Design review of the part built by this model. Coordinates are the model's own, in mm. Coordinates: 2 decimals unless noted, no trailing zeros. Write each loop counter-clockwise with the first axis right and the second up, starting at its lowest first coordinate (ties: lowest second). Pieces come first, ordered by that corner, then holes.
Q1. Add section A-A, the plane x = -51.5. Give the number of separate pieces and of enclosed holes in the cut face, plus the area to 3 significant figures.
Q2. To check wall thickness, follow probe 1 along Y at (x, z) = (-132.5, 1.15); probe 2 along X at (y, z) = (333.5, 0.15); probe 3 along Y at (x, z) = (132.5, 1.25). State the ranges of each line that lie inside material, in increasing order.
Q3. Add section C-C, the plane y = 200.5. Give the boundary of the cut face in (x, z).
Q4. Clearance check with a flat-ended pin moving along its axis: pin 1 Ø0.6 at (y, z) = (333, 1.5) entering from +X. State where the tip first meets the part, or that it passes through.
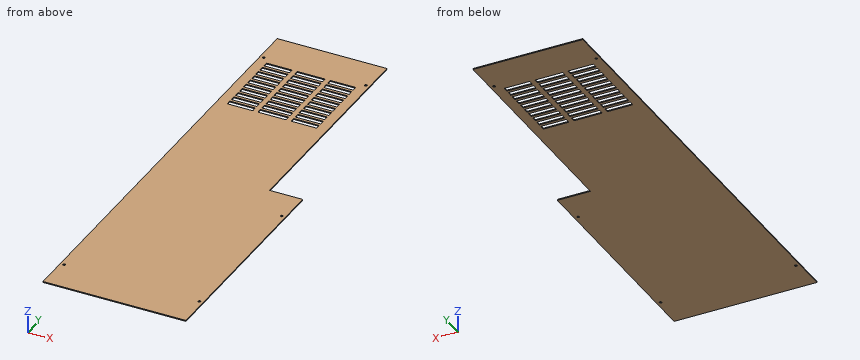
from build123d import *

# Parameters (mm, degrees)
SKETCH_R            = 2.5
PAD_DEPTH           = 2
SKETCH001_W         = 50
SKETCH001_H         = 10
SKETCH001_W_2       = 55
POCKET_DEPTH        = 5
LINEARPATTERN_COUNT = 10
LINEARPATTERN_PITCH = 15.555556


with BuildPart() as part:
    # Sketch → Pad (new body)
    with BuildSketch(Plane.XY):
        Polygon((-140, 447.5), (75, 447.5), (75, -1.5), (140, -1.5), (140, -447.5), (-140, -447.5), align=None)
        with Locations((-132.5, 381.5)):
            Circle(SKETCH_R, mode=Mode.SUBTRACT)
        with Locations((67.5, 381.5)):
            Circle(SKETCH_R, mode=Mode.SUBTRACT)
        with Locations((132.5, -66.5)):
            Circle(SKETCH_R, mode=Mode.SUBTRACT)
        with Locations((132.5, -381.5)):
            Circle(SKETCH_R, mode=Mode.SUBTRACT)
        with Locations((-132.5, -381.5)):
            Circle(SKETCH_R, mode=Mode.SUBTRACT)
    extrude(amount=PAD_DEPTH)

    # Sketch001 → Pocket (cut)
    with BuildSketch(Plane.XY.offset(2)):
        with Locations((-95, 362.5)):
            Rectangle(SKETCH001_W, SKETCH001_H)
        with Locations((30, 362.5)):
            Rectangle(SKETCH001_W, SKETCH001_H)
        with Locations((-32.5, 362.5)):
            Rectangle(SKETCH001_W_2, SKETCH001_H)
    pocket = extrude(amount=-POCKET_DEPTH, mode=Mode.SUBTRACT)

    # LinearPattern: Pocket ×10
    with Locations(*[(0, -i * LINEARPATTERN_PITCH, 0) for i in range(1, LINEARPATTERN_COUNT)]):
        add(pocket, mode=Mode.SUBTRACT)


solid = part.part
Here are the results:
1. separate pieces: 11
1. enclosed holes: 0
1. area: 1,590 mm2
2. probe 1: y = -447.5 to -384, -379 to 379, 384 to 447.5
2. probe 2: x = -140 to -120, -70 to -60, -5 to 5, 55 to 75
2. probe 3: y = -447.5 to -384, -379 to -69, -64 to -1.5
3. outline: (-140, 0) - (75, 0) - (75, 2) - (-140, 2) - close
4. pin 1: stops at x = 75
